Work out the finished part from the listing and answer in its coordinate system (mm). A direction names the side the tool comes from. Give positions to 0.01 mm unless a question says otherwise; leave off trailing zeros. Loops run counter-clockwise (first coordinate to the right, second up) from the corner with the lowest first, then second, coordinate; pieces in that order, holes last. Notation, with made-up numbers: (-2, 82.25) - (51, 82.25) arc R25 ccw to (51, 119.25) - close; hole circle Ø8 at (-21.5, 69.25). An arc over 180 degrees is marked (long way). One line per question, with ' | ' between items.
from build123d import *
from build123d.topology import SkipClean

# Parameters (mm, degrees)
SKETCH1_R                = 43.18
SKETCH1_R_2              = 38.1
SKETCH1_R_3              = 36.195
BOSS_EXTRUDE1_DEPTH      = 2.54
BOSS_EXTRUDE2_START      = 4.318
SKETCH2_R                = 43.18
SKETCH2_R_2              = 40.64
BOSS_EXTRUDE2_DEPTH      = 4.318
SKETCH7_W                = 5.08
SKETCH7_H                = 10.16
CUT_EXTRUDE1_DEPTH       = 12.7
SKETCH12_R               = 43.18
SKETCH12_R_2             = 36.195
BOSS_EXTRUDE3_DEPTH      = 12.192
BOSS_EXTRUDE4_REACH      = 99.671
BOSS_EXTRUDE4_END_RADIUS = 43.18
SKETCH13_W               = 43.18
SKETCH13_H               = 24.13
BOSS_EXTRUDE5_DEPTH      = 38.1
SKETCH14_W               = 38.1
SKETCH14_H               = 19.05
CUT_EXTRUDE2_DEPTH       = 35.56
SKETCH17_R               = 3.2385
CUT_EXTRUDE3_DEPTH       = 35.56


with BuildPart() as part:
    # Sketch1 → Boss-Extrude1 (new body)
    # profile 1 of 2: a face of its own
    with BuildSketch(Plane(origin=(0, 0, 0), x_dir=(1, 0, 0), z_dir=(0, 1, 0))):
        with Locations(Location((0, 0, 0), (0, 0, 270))):
            Circle(SKETCH1_R)
        Circle(SKETCH1_R_2, mode=Mode.SUBTRACT)
    # profile 2 of 2: a face of its own
    with BuildSketch(Plane(origin=(0, 0, 0), x_dir=(1, 0, 0), z_dir=(0, 1, 0))):
        Circle(SKETCH1_R_2)
        with Locations(Location((0, 0, 0), (0, 0, 270))):
            Circle(SKETCH1_R_3, mode=Mode.SUBTRACT)
    extrude(amount=BOSS_EXTRUDE1_DEPTH)

    # Sketch2 → Boss-Extrude2 (add)
    with BuildSketch(Plane.XZ.offset(BOSS_EXTRUDE2_START)):
        with Locations(Location((0, 0, 0), (0, 0, 270))):
            Circle(SKETCH2_R)
        with Locations(Location((0, 0, 0), (0, 0, 270))):
            Circle(SKETCH2_R_2, mode=Mode.SUBTRACT)
    extrude(amount=-BOSS_EXTRUDE2_DEPTH)

    # Sketch3 → Revolve1 (revolve)
    with BuildSketch(Plane.XY, mode=Mode.PRIVATE) as revolve1_sk:
        Polygon((-40.64, -4.318), (-43.18, -4.318), (-43.18, -9.398), (-39.878, -9.398), (-39.878, -6.858), align=None)
    revolve(revolve1_sk.sketch.rotate(Axis((0, 0, 0), (0, 1, 0)), 270), axis=Axis((0, 0, 0), (0, 1, 0)))

    # Sketch7 → Cut-Extrude1 (cut)
    with SkipClean():  # the faces are left unmerged after this step: merging them gives an invalid solid
        with BuildSketch(Plane.XY.offset(43.18)):
            with Locations((-2.54, -5.08)):
                Rectangle(SKETCH7_W, SKETCH7_H)
            with Locations((2.54, -5.08)):
                Rectangle(SKETCH7_W, SKETCH7_H)
        extrude(amount=-CUT_EXTRUDE1_DEPTH, mode=Mode.SUBTRACT)

    # Sketch12 → Boss-Extrude3 (add)
    with SkipClean():  # the faces are left unmerged after this step: merging them gives an invalid solid
        with BuildSketch(Plane(origin=(0, 2.54, 0), x_dir=(1, 0, 0), z_dir=(0, 1, 0))):
            with Locations(Location((0, 0, 0), (0, 0, 263.243672969))):
                Circle(SKETCH12_R)
            with Locations(Location((0, 0, 0), (0, 0, 270))):
                Circle(SKETCH12_R_2, mode=Mode.SUBTRACT)
        extrude(amount=BOSS_EXTRUDE3_DEPTH)

    # Boss-Extrude4: up to this cylinder (the profile starts outside it)
    with SkipClean():  # the faces are left unmerged after this step: merging them gives an invalid solid
        boss_extrude4_end = Plane(origin=(0, 2.667, 0), z_dir=(0, -1, 0)) * Cylinder(BOSS_EXTRUDE4_END_RADIUS, 286.702, mode=Mode.PRIVATE)
        # Sketch8 → Boss-Extrude4 (add, up to the surface)
        with BuildSketch(Plane(origin=(43.18, 0, 0), x_dir=(0, 0, -1), z_dir=(1, 0, 0)), mode=Mode.PRIVATE) as boss_extrude4_sk1:
            Polygon((0.14993237, -9.398), (21.73993237, -9.398), (21.73993237, 14.732), (-21.44006763, 14.732), (-21.44006763, -9.398), align=None)
        boss_extrude4_tool1 = extrude(boss_extrude4_sk1.sketch, amount=-BOSS_EXTRUDE4_REACH, mode=Mode.PRIVATE) - boss_extrude4_end
        add(boss_extrude4_tool1.solids().sort_by_distance((43.18, 2.667, -0.149932))[0])
        add(boss_extrude4_tool1.solids().sort_by_distance((43.18, 2.667, -0.149932))[1])

    # Sketch13 → Boss-Extrude5 (add)
    with SkipClean():  # the faces are left unmerged after this step: merging them gives an invalid solid
        with BuildSketch(Plane(origin=(43.18, 0, 0), x_dir=(0, 0, -1), z_dir=(1, 0, 0))):
            with Locations((0.14993237, 2.667)):
                Rectangle(SKETCH13_W, SKETCH13_H)
        extrude(amount=BOSS_EXTRUDE5_DEPTH)

    # Sketch14 → Cut-Extrude2 (cut)
    with SkipClean():  # the faces are left unmerged after this step: merging them gives an invalid solid
        with BuildSketch(Plane(origin=(81.28, 0, 0), x_dir=(0, 0, -1), z_dir=(1, 0, 0))):
            with Locations((0.14993237, 2.667)):
                Rectangle(SKETCH14_W, SKETCH14_H)
        extrude(amount=-CUT_EXTRUDE2_DEPTH, mode=Mode.SUBTRACT)

    # Sketch17 → Cut-Extrude3 (cut)
    with SkipClean():  # the faces are left unmerged after this step: merging them gives an invalid solid
        with BuildSketch(Plane(origin=(0, 14.732, 0), x_dir=(1, 0, 0), z_dir=(0, 1, 0))):
            with Locations(Location((62.23, 0.14993237, 0), (0, 0, 90))):
                Circle(SKETCH17_R)
        extrude(amount=-CUT_EXTRUDE3_DEPTH, mode=Mode.SUBTRACT)


solid = part.part
1. Find section D-D on z = 0. Write down the section's boundary in (x, y) (3 decimals), then the cut area to 3 significant figures.
Evaluation:
outline: (-43.18, -9.398) - (-39.878, -9.398) - (-39.878, -6.858) - (-40.64, -4.318) - (-40.64, 0) - (-36.195, 0) - (-36.195, 14.732) - (-43.18, 14.732) - close; (36.195, 0) - (40.64, 0) - (40.64, -4.318) - (39.878, -6.858) - (39.878, -9.398) - (58.995, -9.398) - (58.995, -6.858) - (45.72, -6.858) - (45.72, 12.192) - (58.995, 12.192) - (58.995, 14.732) - (36.195, 14.732) - close; (65.465, -9.398) - (81.28, -9.398) - (81.28, -6.858) - (65.465, -6.858) - close; (65.465, 12.192) - (81.28, 12.192) - (81.28, 14.732) - (65.465, 14.732) - close | area: 468 mm2
2. Find section B-B on y = -1.5. Write down the section's boundary in (x, z).
Evaluation:
outline: (-5.08, 40.32) - (-5.08, 42.88) arc R43.18 ccw (long way) to (37.31, -21.74) - (81.28, -21.74) - (81.28, -19.2) - (45.72, -19.2) - (45.72, 18.9) - (81.28, 18.9) - (81.28, 21.44) - (37.48, 21.44) arc R43.18 ccw to (5.08, 42.88) - (5.08, 40.32) arc R40.64 cw (long way) to start
3. Find section C-C on y = 10.25. Write down the section's boundary in (x, z) (3 decimals).
Evaluation:
outline: (37.308, -21.74) - (81.28, -21.74) - (81.28, -19.2) - (45.72, -19.2) - (45.72, 18.9) - (81.28, 18.9) - (81.28, 21.44) - (37.481, 21.44) arc R43.18 ccw (long way) to start; hole circle Ø72.39 at (0, 0)
4. Determine the mould class of faces 4 (the cylindrical face through (59.02, 13.48, 0.27)), 5 (the flat face through (59, 2, -21.74)), 6 (the flat face through (32, 14.732, -19)) for opening direction Z: +Z half, -Z half, draft (parallel to the pull), parting line (faces both ways), or undercut.
Evaluation:
face 4: undercut | face 5: -Z half | face 6: draft
5. Find section A-A on x = 62.23. Write down the section's boundary in (y, z), then the cut area to 3 significant figures.
Evaluation:
outline: (-9.4, -21.74) - (14.73, -21.74) - (14.73, -3.39) - (12.19, -3.39) - (12.19, -19.2) - (-6.86, -19.2) - (-6.86, -3.39) - (-9.4, -3.39) - close; (-9.4, 3.09) - (-6.86, 3.09) - (-6.86, 18.9) - (12.19, 18.9) - (12.19, 3.09) - (14.73, 3.09) - (14.73, 21.44) - (-9.4, 21.44) - close | area: 283 mm2
6. Flat-ended cylindrical pins translate along their axes: pin 1 (2 mm diameter, centred on x = -27, y = -6.5, fed in from -Z); pin 2 (4 mm diameter, centred on y = 6.5, z = -21.5, fed in from -X); pin 3 (12 mm diameter, centred on x = 29, y = 1, fed in from -Z). Find the tip coordinate at first contact, or state that the pin passes through.
Evaluation:
pin 1: z = -34.47 | pin 2: x = -38.53 | pin 3: z = -36.54
7. Consider L1, parallel to Z at x = 47, y = -6.5; L2, parallel to Y at x = 55.5, z = -15; L3, parallel to Z at x = 62.23, y = 13.55. Determine where each line is inside the solid, lowest interval first.
Evaluation:
L1: -21.74 to -19.2, 18.9 to 21.44 | L2: -9.4 to -6.86, 12.19 to 14.73 | L3: -21.74 to -3.39, 3.09 to 21.44
8. Which of the six approach directions +Z, -Z, +X, -X, +Y, -Y give full straight-line access (tool end or side, diameter ignored) to faces 1 (the flat face through (59, 2, 21.44)), 2 (the flat face through (45.72, 3, 0)), 3 (the flat face through (5.08, -5, 42))?
Evaluation:
face 1: +Z, +X, +Y, -Y | face 2: +X | face 3: +Z, -Y
